Source: CAD feature listing. Evaluate the final solid. Frame: model axes, mm. Give positions to 0.01 mm unless a question says otherwise; leave off trailing zeros. Order: outer loops, then holes, each group sorted by start corner. A loop starts at its lowest first (then second) coordinate and runs counter-clockwise, first axis right, second up. Notation, with made-up numbers: M -18,28.25 L 13,28.25 A34 cw 13,58.25 Z; hole C -24,-23.75 d1. An arc over 180 degrees is marked long. Answer in a Markdown table with one row per item. Add a question column.
(1) Section query A-A, the plane z = 0.8. Count the separate pieces of the cut face and the enclosed holes in it, plus the area to 3 significant figures.
(2) Section query B-B, the plane y = -203. Return loops of the section in (x, z).
(3) Material intervals for line 1 along X through (y, z) = (-16, 0.8); line 2 along X through (y, z) = (12, 1.15); line 3 along Y through (x, z) = (109, 1), sorted ascending.
(4) Pin query (flat end, axial travel): P1, Ø0.5, axis at x = -668, z = 1, coming from the +Y side; P2, Ø0.8, axis at x = -645, z = 0.5, coming from the +Y side. Return the tip coordinate at first contact, or that it passes through.
from build123d import *

# Parameters (mm, degrees)
F0_W     = 26.9875
F0_H     = 19.05
F0_W_2   = 327.025
F0_H_2   = 76.2
F0_W_3   = 12.7
F0_H_3   = 50.8
F1_DEPTH = 1.651
F2_R     = 12.7
F3_R     = 3.175
F4_R     = 12.7


with BuildPart() as f1:
    # F0 (on Top) → F1 (new body)
    with BuildSketch(Plane.XY):
        Polygon((-651.0655, -152.4), (-651.0655, -101.6), (-651.0655, -87.3125), (-678.053, -87.3125), (-678.053, -166.6875), (-651.0655, -166.6875), align=None)
        Polygon((638.3655, 254), (-638.3655, 254), (-638.3655, 152.4), (-638.3655, 101.6), (-638.3655, 25.4), (-638.3655, -25.4), (-638.3655, -101.6), (-638.3655, -152.4), (-638.3655, -254), (638.3655, -254), (695.1345, -254), (695.1345, 254), align=None)
        with Locations((630.84075, -146.05)):
            Rectangle(F0_W, F0_H, mode=Mode.SUBTRACT)
        with Locations((630.84075, -107.95)):
            Rectangle(F0_W, F0_H, mode=Mode.SUBTRACT)
        with Locations((630.84075, -19.05)):
            Rectangle(F0_W, F0_H, mode=Mode.SUBTRACT)
        with Locations((0, 95.25)):
            Rectangle(F0_W_2, F0_H_2, mode=Mode.SUBTRACT)
        with Locations((630.84075, 19.05)):
            Rectangle(F0_W, F0_H, mode=Mode.SUBTRACT)
        with Locations((630.84075, 107.95)):
            Rectangle(F0_W, F0_H, mode=Mode.SUBTRACT)
        with Locations((630.84075, 146.05)):
            Rectangle(F0_W, F0_H, mode=Mode.SUBTRACT)
        with Locations((-644.7155, -127)):
            Rectangle(F0_W_3, F0_H_3)
        Polygon((-651.0655, 101.6), (-651.0655, 152.4), (-651.0655, 166.6875), (-678.053, 166.6875), (-678.053, 87.3125), (-651.0655, 87.3125), align=None)
        with Locations((-644.7155, 0)):
            Rectangle(F0_W_3, F0_H_3)
        Polygon((-651.0655, -25.4), (-651.0655, 25.4), (-651.0655, 39.6875), (-678.053, 39.6875), (-678.053, -39.6875), (-651.0655, -39.6875), align=None)
        with Locations((-644.7155, 127)):
            Rectangle(F0_W_3, F0_H_3)
    extrude(amount=F1_DEPTH)

    # F2
    f2_edges = [f1.edges().sort_by_distance(p)[0] for p in [
        (-163.5125, 133.35, 0.8255),
        (163.5125, 133.35, 0.8255),
        (-163.5125, 57.15, 0.8255),
        (163.5125, 57.15, 0.8255),
    ]]
    fillet(f2_edges, radius=F2_R)

    # F3
    f3_edges = [f1.edges().sort_by_distance(p)[0] for p in [
        (-678.053, 166.6875, 0.8255),
        (-651.0655, 166.6875, 0.8255),
        (-638.3655, 152.4, 0.8255),
        (-651.0655, 152.4, 0.8255),
        (-651.0655, 87.3125, 0.8255),
        (-651.0655, 101.6, 0.8255),
        (-678.053, 87.3125, 0.8255),
        (-638.3655, 101.6, 0.8255),
        (-638.3655, -25.4, 0.8255),
        (-638.3655, 25.4, 0.8255),
        (-651.0655, 39.6875, 0.8255),
        (-651.0655, 25.4, 0.8255),
        (-678.053, 39.6875, 0.8255),
        (-678.053, -39.6875, 0.8255),
        (-651.0655, -39.6875, 0.8255),
        (-651.0655, -25.4, 0.8255),
        (-638.3655, -101.6, 0.8255),
        (-651.0655, -87.3125, 0.8255),
        (-678.053, -87.3125, 0.8255),
        (-678.053, -166.6875, 0.8255),
        (-651.0655, -166.6875, 0.8255),
        (-638.3655, -152.4, 0.8255),
        (-651.0655, -152.4, 0.8255),
        (617.347, 155.575, 0.8255),
        (617.347, 117.475, 0.8255),
        (617.347, 28.575, 0.8255),
        (617.347, -136.525, 0.8255),
        (617.347, -98.425, 0.8255),
        (617.347, -9.525, 0.8255),
        (617.347, 9.525, 0.8255),
        (617.347, -28.575, 0.8255),
        (617.347, -117.475, 0.8255),
        (617.347, -155.575, 0.8255),
        (644.3345, -155.575, 0.8255),
        (644.3345, -136.525, 0.8255),
        (644.3345, -98.425, 0.8255),
        (644.3345, 155.575, 0.8255),
        (644.3345, 117.475, 0.8255),
        (644.3345, 98.425, 0.8255),
        (644.3345, 9.525, 0.8255),
        (644.3345, 136.525, 0.8255),
        (644.3345, -28.575, 0.8255),
        (644.3345, 28.575, 0.8255),
        (644.3345, -117.475, 0.8255),
    ]]
    fillet(f3_edges, radius=F3_R)

    # F4
    f4_edges = [f1.edges().sort_by_distance(p)[0] for p in [
        (695.1345, 254, 0.8255),
        (695.1345, -254, 0.8255),
        (-638.3655, -254, 0.8255),
        (-638.3655, 254, 0.8255),
    ]]
    fillet(f4_edges, radius=F4_R)


solid = f1.part
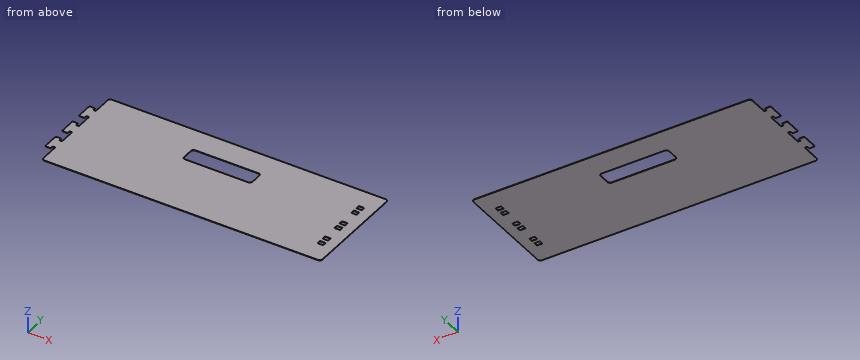
Values follow:
| question | item | result |
|---|---|---|
| 1 | separate pieces | 1 |
| 1 | enclosed holes | 7 |
| 1 | area | 658,000 mm² |
| 2 | outline | M -638.37,0 L 695.13,0 L 695.13,1.65 L -638.37,1.65 Z |
| 3 | line 1 | x = -678.05 to 617.35, 644.33 to 695.13 |
| 3 | line 2 | x = -678.05 to 617.43, 644.26 to 695.13 |
| 3 | line 3 | y = -254 to 57.15, 133.35 to 254 |
| 4 | P1 | stops at y = 166.69 |
| 4 | P2 | stops at y = 152.4 |
